CAD build for the part. Positions are in the model's coordinates, mm. Face numbers are marked on the shaded views. A direction names the side the tool comes from. Give positions to 0.01 mm unless a question says otherwise; leave off trailing zeros. Loops run counter-clockwise (first coordinate to the right, second up) from the corner with the lowest first, then second, coordinate; pieces in that order, holes last. Notation, with made-up numbers: M -33,70.5 L 3,70.5 A9 ccw 3,74.5 Z; hole C 47,81 d8. An arc over 180 degrees is marked long. Answer as CSV lines item,"result".
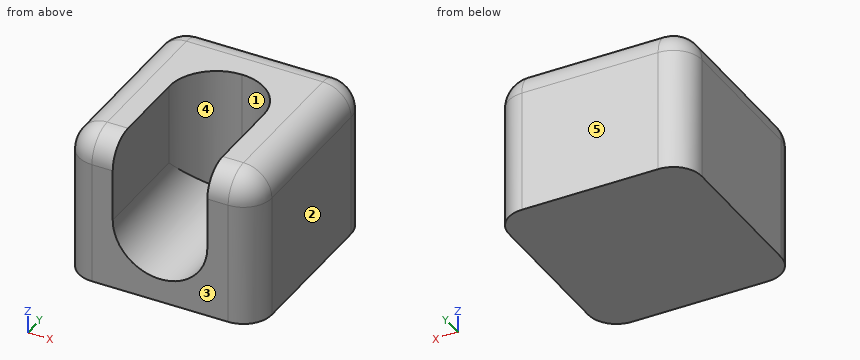
from build123d import *

# Parameters (mm, degrees)
SKETCH1_W      = 20.4
SKETCH1_H      = 21.5
EXTRUDE1_DEPTH = 16
FILLET8_R      = 3
SKETCH2_W      = 14.5
SKETCH2_H      = 17
EXTRUDE2_DEPTH = 5
FILLET9_R      = 5
FILLET10_R     = 5


# Some blends are built 0.0001 mm under size
with BuildPart() as part:
    # Sketch1 → Extrude1 (new body)
    with BuildSketch(Plane.XY):
        with Locations((10.2, 10.75)):
            Rectangle(SKETCH1_W, SKETCH1_H)
    extrude(amount=-EXTRUDE1_DEPTH)

    # Fillet8
    fillet8_edges = [part.edges().sort_by_distance(p)[0] for p in [
        (10.2, 21.5, 0),
        (20.4, 10.75, 0),
        (10.2, 0, 0),
        (0, 10.75, 0),
        (0, 21.5, -8),
        (20.4, 21.5, -8),
        (20.4, 0, -8),
        (0, 0, -8),
    ]]
    fillet(fillet8_edges, radius=FILLET8_R)

    # Sketch2 → Extrude2 (cut, symmetric)
    with BuildSketch(Plane(origin=(10.2, 0, 0), x_dir=(0, 0, -1), z_dir=(1, 0, 0))):
        with Locations((6.25, 7.5)):
            Rectangle(SKETCH2_W, SKETCH2_H)
    extrude(amount=EXTRUDE2_DEPTH, both=True, mode=Mode.SUBTRACT)

    # Fillet9
    fillet9_edges = [part.edges().sort_by_distance(p)[0] for p in [
        (5.2, 16, -6.75),
        (15.2, 16, -6.75),
    ]]
    fillet(fillet9_edges, radius=FILLET9_R - 0.0001)  # a hair under: the kernel refuses the full size

    # Fillet10
    # the kernel refuses this fillet: 5 mm, written as the material it adds along each edge
    with BuildSketch(Plane(origin=(5.2, 23.5001, -13.5), x_dir=(0, 0, 1), z_dir=(0, -1, 0))) as fillet10_piece_1_section:
        with BuildLine():
            CenterArc((FILLET10_R, -FILLET10_R), FILLET10_R, 90, 90)
            Line((0, -FILLET10_R), (0, 0))
            Line((0, 0), (FILLET10_R, 0))
        make_face()
    fillet10_piece_1 = extrude(amount=23.5001, mode=Mode.PRIVATE)
    fillet10_piece_1 = split(fillet10_piece_1, bisect_by=Plane(origin=(6.690730553, 21.5, -12.634344102), z_dir=(0, -1, 0)), keep=Keep.TOP, mode=Mode.PRIVATE)
    add(fillet10_piece_1)
    with BuildSketch(Plane(origin=(15.2, 23.5001, -13.5), x_dir=(-1, 0, 0), z_dir=(0, -1, 0))) as fillet10_piece_2_section:
        with BuildLine():
            CenterArc((FILLET10_R, -FILLET10_R), FILLET10_R, 90, 90)
            Line((0, -FILLET10_R), (0, 0))
            Line((0, 0), (FILLET10_R, 0))
        make_face()
    fillet10_piece_2 = extrude(amount=23.5001, mode=Mode.PRIVATE)
    fillet10_piece_2 = split(fillet10_piece_2, bisect_by=Plane(origin=(13.709267183, 21.5, -12.634319822), z_dir=(0, -1, 0)), keep=Keep.TOP, mode=Mode.PRIVATE)
    add(fillet10_piece_2)


solid = part.part
1) Band-saw the part on C-C on x = 6.5. Give the cut face in (y, z).
Answer below:
outline,"M 0,-16 L 21.5,-16 L 21.5,-3 A3 ccw 18.5,0 L 14.36,0 L 14.36,-11.86 L 0,-11.86 Z"
2) Which spindle directions (+Z, -Z, +X, -X, +Y, -Y) get a long thin tool onto all of the face, cutting with end or side? Do the marked faces 4 and 5. Say none if no direction does.
Answer below:
face 4,"+Z, -Y"
face 5,"+Z, -Z, +X, -X, +Y"
3) Drill centre lines: line 1 (X direction, y = 10.75, z = -4.75); line 2 (Y direction, x = 10.25, z = -3.25); line 3 (Z direction, x = 17.5, y = 6.25). Where is each one in solid material? Low to high. Write a range as from..to.
Answer below:
line 1,"x = 0..5.2, 15.2..20.4"
line 2,"y = 16..21.5"
line 3,"z = -16..0"
4) Flat gauge pins, fed straight in: pin 1 (4 mm diameter, centred on x = 12, y = 2.5, fed in from +Z); pin 2 (7 mm diameter, centred on y = 6.5, z = -2.5, fed in from +X). Where does each tip first touch, or does it go through?
Answer below:
pin 1,"stops at z = -11.75"
pin 2,"stops at x = 20.4"
5) Band-saw the part on A-A on y = 7.5. Give the cut face in (x, z).
Answer below:
outline,"M 0,-16 L 20.4,-16 L 20.4,-3 A3 ccw 17.4,0 L 15.2,0 L 15.2,-8.5 A5 cw 5.2,-8.5 L 5.2,0 L 3,0 A3 ccw 0,-3 Z"
6) Mould opens along X. For the marked faces 1, 2 and 3 say: +X half, -X half, draft (parallel to the pull), parting line (faces both ways), or undercut.
Answer below:
face 1,"undercut"
face 2,"+X half"
face 3,"draft"
7) Band-saw the part on B-B on z = -14.25. Give the cut face in (x, y), and give its area (3 significant figures).
Answer below:
outline,"M 0,3 A3 ccw 3,0 L 17.4,0 A3 ccw 20.4,3 L 20.4,18.5 A3 ccw 17.4,21.5 L 3,21.5 A3 ccw 0,18.5 Z"
area,"431 mm^2"
